Check sheet for the drawn part. Datum: minimum x, y, z corner. Units: mm. A direction names the side the tool comes from. Round coordinates to 2 decimals unless told otherwise and drop trailing zeros. Write each loop counter-clockwise with the first axis right and the second up, starting at its lowest first coordinate (ties: lowest second). Pieces come first, ordered by that corner, then holes.
Item 1: Release check for a two-part mould opening along X. For the marked faces 1, 2 and 3 record: +X half, -X half, draft (parallel to the pull), parting line (faces both ways), or undercut.
Item 2: Tool access check on the marked faces 4 and 5. Record the directions out of +Z, -Z, +X, -X, +Y, -Y that give a thin tool (end or side, any length) a straight path to the whole face; none if there is none.
Item 3: Cross-section at B-B on z = 16.5. Enter the section's corners in (x, y).
Item 4: Cross-section at C-C on x = 10. Enter the section's corners in (y, z).
Item 5: Material ranges on line 1 (X direction, y = 3.75, z = 9.5); line 2 (Y direction, x = 6.75, z = 27.5); line 3 (X direction, y = 0.5, z = 12), recorded low to high.
Item 6: Cross-section at A-A on y = 3. Enter the section's corners in (x, z).
Item 7: Go/stop test with flat-tipped pins: pin 1 Ø2.5 at (y, z) = (3.5, 28.5) entering from +X; pin 2 Ø1.5 at (x, z) = (9, 27.5) entering from +Y; pin 3 Ø2.5 at (x, z) = (10.5, 28) entering from -Y. Record where each tip stops, or that it passes through.
Item 8: Cross-section at D-D on x = 3. Enter the section's corners in (y, z).
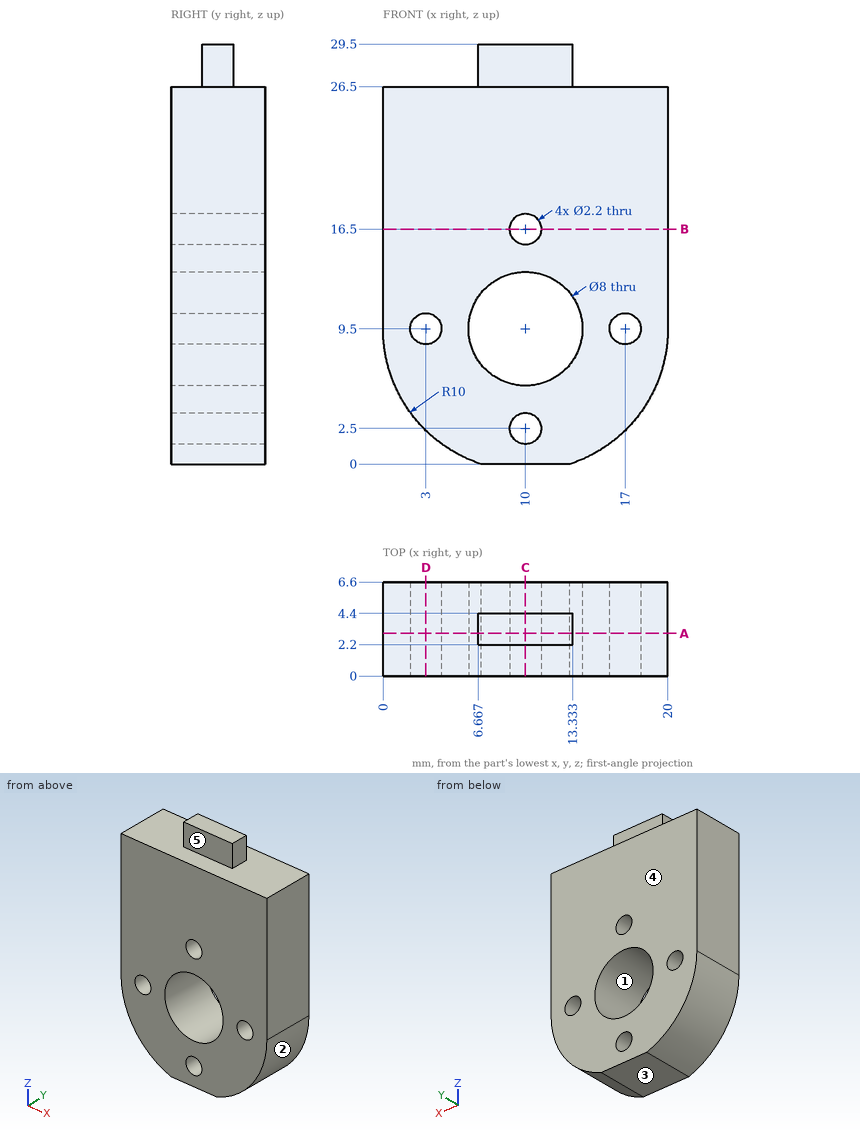
Response values:
1. face 1: undercut
1. face 2: +X half
1. face 3: draft
2. face 4: +Z, -Z, +X, -X, +Y
2. face 5: +Z, +X, -X, -Y
3. outline: (0, 0) - (8.9, 0) - (8.9, 6.6) - (0, 6.6) - close; (11.1, 0) - (20, 0) - (20, 6.6) - (11.1, 6.6) - close
4. outline: (0, 0) - (6.6, 0) - (6.6, 1.4) - (0, 1.4) - close; (0, 3.6) - (6.6, 3.6) - (6.6, 5.5) - (0, 5.5) - close; (0, 13.5) - (6.6, 13.5) - (6.6, 15.4) - (0, 15.4) - close; (0, 17.6) - (6.6, 17.6) - (6.6, 26.5) - (4.4, 26.5) - (4.4, 29.5) - (2.2, 29.5) - (2.2, 26.5) - (0, 26.5) - close
5. line 1: x = 0 to 1.9, 4.1 to 6, 14 to 15.9, 18.1 to 20
5. line 2: y = 2.2 to 4.4
5. line 3: x = 0 to 6.88, 13.12 to 20
6. outline: (0, 9.5) arc R10 ccw to (6.88, 0) - (13.12, 0) arc R10 ccw to (20, 9.5) - (20, 26.5) - (13.33, 26.5) - (13.33, 29.5) - (6.67, 29.5) - (6.67, 26.5) - (0, 26.5) - close; hole circle Ø2.2 at (3, 9.5); hole circle Ø8 at (10, 9.5); hole circle Ø2.2 at (10, 2.5); hole circle Ø2.2 at (10, 16.5); hole circle Ø2.2 at (17, 9.5)
7. pin 1: stops at x = 13.33
7. pin 2: stops at y = 4.4
7. pin 3: stops at y = 2.2
8. outline: (0, 2.36) - (6.6, 2.36) - (6.6, 8.4) - (0, 8.4) - close; (0, 10.6) - (6.6, 10.6) - (6.6, 26.5) - (0, 26.5) - close
